Input: part model. Units: mm. Frame: model coordinates. Round coordinates to 2 decimals unless told otherwise and drop trailing zeros. Loops run counter-clockwise (first coordinate to the right, second up) from the corner with the lowest first, then second, coordinate; pieces in that order, holes last. Notation, with made-up numbers: (-2.5, 62) - (32.5, 62) arc R12 ccw to (32.5, 70) - close; hole circle Ø10 at (57.25, 54.25). An arc over 180 degrees is marked (long way). Write each question's results on one line, items separated by ' | '.
Autodesk Fusion 360 part; units mm, degrees
sketch "Sketch1" plane through (0, 0, 0) normal (0, 1, 0) x (1, 0, 0)
  arc A0 (12.5, 96.75) -> (-12.5, 96.75) centre (0, 96.75) ccw
  line L0 (12.5, 96.75) -> (12.5, 10.75)
  arc A1 (-12.5, 10.75) -> (12.5, 10.75) centre (0, 10.75) ccw
  circle A2 centre (0, 96.75) radius 3
  circle A3 centre (0, 10.75) radius 3
  line L1 (-12.5, 10.75) -> (-12.5, 96.75)
extrude "Extrude1" add sketch "Sketch1" along normal blind 6
1. Section query B-B, the plane y = 3.4. Output: boundary loops of the cut face in (x, z).
Answer:
outline: (-12.5, -96.75) arc R12.5 ccw to (12.5, -96.75) - (12.5, -10.75) arc R12.5 ccw to (-12.5, -10.75) - close; hole circle Ø6 at (0, -96.75); hole circle Ø6 at (0, -10.75)
2. Section query D-D, the plane x = 4.5. Output: boundary loops of the cut face in (y, z), plus the area to 3 significant figures.
Answer:
outline: (0, -108.41) - (6, -108.41) - (6, 0.91) - (0, 0.91) - close | area: 656 mm^2
3. Mould query, pull axis X, two halves, no side actions, for faces 1 (the flat face through (0, 0, -55)), 2 (the cylindrical face through (-0.65, 2.96, -99.68)), 3 (the flat face through (12.5, 3, -54)), 4 (the cylindrical face through (-0.275, 2.958, -109.247)). Classes: pulls with the +X half, pulls with the -X half, needs draft (parallel to the pull), parting line crosses it, or undercut.
Answer:
face 1: needs draft | face 2: undercut | face 3: pulls with the +X half | face 4: parting line crosses it
4. Section query C-C, the plane x = 10. Output: boundary loops of the cut face in (y, z), plus the area to 3 significant figures.
Answer:
outline: (0, -104.25) - (6, -104.25) - (6, -3.25) - (0, -3.25) - close | area: 606 mm^2
5. Contact query for flat-ended pins moving along their axis: pin 1 (1.5 mm diameter, centred on x = 4, y = 1, fed in from -Z); pin 2 (5.5 mm diameter, centred on x = 0, z = -10.75, fed in from +Y). Output: stop coordinate, or through.
Answer:
pin 1: z = -108.82 | pin 2: through
6. Line query: line 1 (Z direction, x = 0, y = 4); line 2 (X direction, y = 3.75, z = -10.75); line 3 (X direction, y = 3.45, z = -100.5). Output: solid intervals per line, ascending. Write a range as [from, to].
Answer:
line 1: [-109.25, -99.75], [-93.75, -13.75], [-7.75, 1.75] | line 2: [-12.5, -3], [3, 12.5] | line 3: [-11.92, 11.92]
7. Section query A-A, the plane x = 0. Output: boundary loops of the cut face in (y, z), plus the area to 3 significant figures.
Answer:
outline: (0, -109.25) - (6, -109.25) - (6, -99.75) - (0, -99.75) - close; (0, -93.75) - (6, -93.75) - (6, -13.75) - (0, -13.75) - close; (0, -7.75) - (6, -7.75) - (6, 1.75) - (0, 1.75) - close | area: 594 mm^2
